Verification items for the finished model (mm, model axes). Face numbers are marked on the shaded views. A direction names the side the tool comes from. Coordinates: 2 decimals unless noted, no trailing zeros. Order: outer loops, then holes, each group sorted by start corner. A loop starts at its lowest first (then second) coordinate and runs counter-clockwise, first axis right, second up. Notation, with made-up numbers: (14, 67) -> (44, 67) arc R22 cw to (44, 74) -> close; hole circle Ø9 at (7, 54.5). An arc over 180 degrees is marked (long way). Answer as CSV lines item,"result".
```python
from build123d import *

# Parameters (mm, degrees)
BOSS_EXTRUDE1_DEPTH = 100
CUT_EXTRUDE1_DEPTH  = 100
CUT_EXTRUDE2_DEPTH  = 100


with BuildPart() as part:
    # Sketch1 → Boss-Extrude1 (new body)
    with BuildSketch(Plane.XY):
        Polygon((150, 0), (75, 129.903810568), (-75, 129.903810568), (-150, 0), (-75, -129.903810568), (75, -129.903810568), align=None)
    extrude(amount=-BOSS_EXTRUDE1_DEPTH)

    # Sketch2 → Cut-Extrude1 (cut)
    with BuildSketch(Plane.XY):
        Polygon((-120, 0), (-119.097636783, -1.562938939), (120, 0), (60, 103.923048454), (-60, 103.923048454), align=None)
    extrude(amount=-CUT_EXTRUDE1_DEPTH, mode=Mode.SUBTRACT)

    # Sketch3 → Cut-Extrude2 (cut)
    with BuildSketch(Plane(origin=(0.005127388, -0.784385247, 0), x_dir=(0.9999786356570095, 0.006536683375074496, 0), z_dir=(-0.006536683375074496, 0.9999786356570095, 0))):
        with BuildLine():
            Line((0.446063751, 75), (-49.553936249, 75))
            ThreePointArc((-49.553936249, 75), (-74.553936249, 50), (-49.553936249, 25))
            Line((-49.553936249, 25), (0.446063751, 25))
            ThreePointArc((0.446063751, 25), (-24.553936249, 50), (0.446063751, 75))
        make_face()
        with BuildLine():
            Line((0.446063751, 25), (0.446063751, 75))
            ThreePointArc((0.446063751, 75), (-24.553936249, 50), (0.446063751, 25))
        make_face()
        with BuildLine():
            ThreePointArc((0.446063751, 25), (25.446063751, 50), (0.446063751, 75))
            Line((0.446063751, 75), (0.446063751, 25))
        make_face()
        with BuildLine():
            ThreePointArc((0.446063751, 25), (25.446063751, 50), (0.446063751, 75))
            Line((0.446063751, 75), (50.446063751, 75))
            ThreePointArc((50.446063751, 75), (75.446063751, 50), (50.446063751, 25))
            Line((50.446063751, 25), (0.446063751, 25))
        make_face()
    extrude(amount=-CUT_EXTRUDE2_DEPTH, mode=Mode.SUBTRACT)


solid = part.part
```
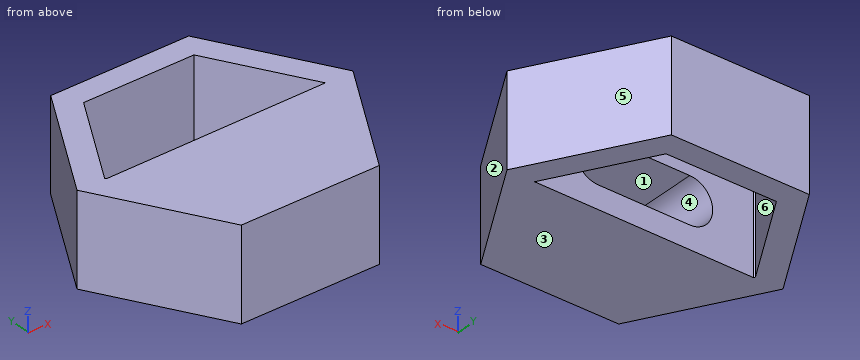
Item 1: Tool access check on the marked faces 4, 5 and 6. Record the directions out of +Z, -Z, +X, -X, +Y, -Y that give a thin tool (end or side, any length) a straight path to the whole face; none if there is none.
Answer list:
face 4,"none"
face 5,"+Z, -Z, +X, +Y"
face 6,"+Z, -Z"
Item 2: Depth check by flat-ended pin: pin 1 Ø12 at (y, z) = (-26.5, -63) entering from -X; pin 2 Ø5 at (x, y) = (94.5, 80) entering from +Z; pin 3 Ø6 at (x, z) = (-96.5, -44.5) entering from -Y; pin 4 Ø2 at (y, z) = (32, -39) entering from -X. Enter the tip coordinate at first touch or a pass-through.
Answer list:
pin 1,"x = -138.16"
pin 2,"z = 0"
pin 3,"y = -97.86"
pin 4,"x = -132.1"
Item 3: Section check D-D, the plane z = -42. Record the boundary of the cut face in (x, y).
Answer list:
outline,"(-150, 0) -> (-75, -129.9) -> (75, -129.9) -> (150, 0) -> (75, 129.9) -> (-75, 129.9) -> close; hole (-120, 0) -> (-119.1, -1.56) -> (-73.23, -1.26) -> (-72.58, -101.26) -> (74.79, -100.3) -> (74.14, -0.3) -> (120, 0) -> (60, 103.92) -> (-60, 103.92) -> close"
Item 4: Section check A-A, the plane z = -6.5. Record the boundary of the cut face in (x, y), plus the area to 3 significant figures.
Answer list:
outline,"(-150, 0) -> (-75, -129.9) -> (75, -129.9) -> (150, 0) -> (75, 129.9) -> (-75, 129.9) -> close; hole (-120, 0) -> (-119.1, -1.56) -> (120, 0) -> (60, 103.92) -> (-60, 103.92) -> close"
area,"39,600 mm2"
Item 5: Release check for a two-part mould opening along Z. For the marked faces 1, 2 and 3 record: +Z half, -Z half, draft (parallel to the pull), parting line (faces both ways), or undercut.
Answer list:
face 1,"undercut"
face 2,"draft"
face 3,"-Z half"
Item 6: Section check C-C, the plane y = 84. Record the boundary of the cut face in (x, z).
Answer list:
outline,"(-101.5, -100) -> (-71.5, -100) -> (-71.5, 0) -> (-101.5, 0) -> close; (71.5, -100) -> (101.5, -100) -> (101.5, 0) -> (71.5, 0) -> close"
Item 7: Thickness scan on line 1 (Y direction, x = 45, z = -94.5); line 2 (Y direction, x = -58.5, z = -71); line 3 (Z direction, x = -54.5, y = -85.5). Record the ranges inside material, lowest first.
Answer list:
line 1,"-129.9 to -0.49, 103.92 to 129.9"
line 2,"-129.9 to -101.17, 103.92 to 129.9"
line 3,"-100 to -74.39, -25.61 to 0"
Item 8: Section check B-B, the plane x = 31.5. Record the boundary of the cut face in (y, z), plus the area to 3 significant figures.
Answer list:
outline,"(-129.9, -100) -> (-0.58, -100) -> (-0.58, -75) -> (-100.58, -75) -> (-100.58, -25) -> (-0.58, -25) -> (-0.58, 0) -> (-129.9, 0) -> close; (103.92, -100) -> (129.9, -100) -> (129.9, 0) -> (103.92, 0) -> close"
area,"10,500 mm2"
